Read the model definition and answer for the solid it produces. Units are mm, in the model's axes. A direction names the side the tool comes from. Coordinates: 2 decimals unless noted, no trailing zeros. Write each loop counter-clockwise with the first axis right and the second up, starting at its lowest first coordinate (ties: lowest second). Pieces come first, ordered by that corner, then holes. Notation, with made-up numbers: (-1, 75.25) -> (7, 75.25) arc R5 cw to (7, 81.25) -> close; hole circle Ø3 at (-11.5, 52). An arc over 180 degrees is marked (long way). Use CSV: the item, a comma, the result in double quotes.
from build123d import *

# Parameters (mm, degrees)
BOSS_EXTRUDE1_DEPTH     = 225
CUT_EXTRUDE2_DEPTH      = 231.295675755
CUT_EXTRUDE2_DEPTH_BACK = 231.295675755
CUT_EXTRUDE3_DEPTH      = 231.06363453
CUT_EXTRUDE3_DEPTH_BACK = 231.06363453


with BuildPart() as part:
    # Sketch1 → Boss-Extrude1 (new, symmetric)
    with BuildSketch(Plane.XY):
        Polygon((-17.90633676, 20.183505355), (-17.90633676, -22.316494645), (-15.40633676, -22.316494645), (-15.40633676, 17.683505355), (24.59366324, 17.683505355), (24.59366324, 20.183505355), align=None)
    extrude(amount=BOSS_EXTRUDE1_DEPTH, both=True)

    # Sketch2 → Cut-Extrude2 (cut, two sides: drawn at the far end of the back side and taken through both)
    with BuildSketch(Plane(origin=(0, 20.183505355, 0), x_dir=(1, 0, 0), z_dir=(0, 1, 0)).offset(-CUT_EXTRUDE2_DEPTH_BACK)):
        Polygon((24.59366324, 182.5), (24.59366324, 225), (-17.90633676, 225), align=None)
        Polygon((24.59366324, -225), (-17.90633676, -225), (24.59366324, -182.5), align=None)
    extrude(amount=CUT_EXTRUDE2_DEPTH + CUT_EXTRUDE2_DEPTH_BACK, mode=Mode.SUBTRACT)

    # Sketch3 → Cut-Extrude3 (cut, two sides: drawn at the far end of the back side and taken through both)
    with BuildSketch(Plane.ZY.offset(17.90633676).offset(-CUT_EXTRUDE3_DEPTH_BACK)):
        Polygon((-225, 20.183505355), (-182.5, -22.316494645), (-225, -22.316494645), align=None)
        Polygon((182.5, -22.316494645), (225, -22.316494645), (225, 20.183505355), align=None)
    extrude(amount=CUT_EXTRUDE3_DEPTH + CUT_EXTRUDE3_DEPTH_BACK, mode=Mode.SUBTRACT)


solid = part.part
1. A tool of negligible diameter and unlimited length cuts with its end or side. For faces 1 (the flat face through (4, 17.684, 3)), 2 (the flat face through (-16.639, -0.769, -204.047)), from which of +Z, -Z, +X, -X, +Y, -Y can it reach the whole face along a straight path? Write none if from no direction.
Solutions:
face 1,"+Z, -Z, +X, -Y"
face 2,"-Z, +X, -X, -Y"
2. This flat-tipped pin is pushed along its axis until it touches: pin 1 Ø4 at (x, z) = (7.5, 125) entering from -Y. Where does it stop, or does it pass through?
Solutions:
pin 1,"stops at y = 17.68"
3. A cutting plane is placed at C-C (x = 15.5). Give the vertices of the cut face in (y, z), and give its area (3 significant figures).
Solutions:
outline,"(17.68, -191.59) -> (20.18, -191.59) -> (20.18, 191.59) -> (17.68, 191.59) -> close"
area,"958 mm^2"
4. A cutting plane is placed at B-B (y = -7). Give the vertices of the cut face in (x, z).
Solutions:
outline,"(-17.91, -197.82) -> (-15.41, -197.82) -> (-15.41, 197.82) -> (-17.91, 197.82) -> close"
5. A cutting plane is placed at A-A (z = -90). Give the vertices of the cut face in (x, y).
Solutions:
outline,"(-17.91, -22.32) -> (-15.41, -22.32) -> (-15.41, 17.68) -> (24.59, 17.68) -> (24.59, 20.18) -> (-17.91, 20.18) -> close"
6. Find the intervals of material crossed by line 1 along X through (y, z) = (15.5, -54); line 2 along Y through (x, z) = (21.5, 77.5); line 3 along Z through (x, y) = (1, 18.5), in increasing order.
Solutions:
line 1,"x = -17.91 to -15.41"
line 2,"y = 17.68 to 20.18"
line 3,"z = -206.09 to 206.09"
